Could you check a few things on this model? Use its own coordinates, in mm. A direction names the side the tool comes from. Coordinates: 2 decimals unless noted, no trailing zeros. Loops run counter-clockwise (first coordinate to the right, second up) from the corner with the lowest first, then second, coordinate; pieces in that order, holes last. Notation, with made-up numbers: (-6, 84.25) - (39, 84.25) arc R20 ccw to (39, 93.25) - close; hole circle Ø5 at (32, -15.75). An arc over 180 degrees is marked (long way). One line per question, with ' | ' between items. Start each with the question number.
1. Please list where these lines run through material, in increasing order: L1, parallel to Z at x = 0, y = 7.25; L2, parallel to Y at x = 0, z = 10.5; L3, parallel to Z at x = -1, y = 6. Write a range as [from, to].
2. Which directions (+Z, -Z, +X, -X, +Y, -Y) give clear straight access to the entire face, cutting with the end or side of a thin tool? Please do faces 1 (the cylindrical face through (1.43, -6.15, 19.45)), 2 (the cylindrical face through (3.958, 1.247, 19.591)).
3. I want a section at A-A, the plane y = 0. Write out the boundary of the cut face in (x, z), then the cut area to 3 significant figures.
4. I want a section at C-C, the plane z = 7. Write out the boundary of the cut face in (x, y), then the cut area to 3 significant figures.
5. I want a section at D-D, the plane y = 3. Write out the boundary of the cut face in (x, z), then the cut area to 3 significant figures.
6. I want a section at B-B, the plane x = 0. Write out the boundary of the cut face in (y, z).
7. We'd pull the mould along Z, two halves only. Please class faces 3 (the flat face through (2, -2, 13)), 4 (the cylindrical face through (-1.5, 5.17, 7.07)), 5 (the flat face through (2, -2, 0)): pulls with the +Z half, pulls with the -Z half, needs draft (parallel to the pull), parting line crosses it, or undercut.
8. I'm going to push flat-ended pins straight in: P1, Ø10, axis at x = 6.5, z = 14, coming from the -Y side; P2, Ø1, axis at x = -1, z = 22.5, coming from the +Y side; P3, Ø4, axis at y = 2.5, z = 13.5, coming from the +X side. Where does each tip first touch, or does it pass through?
from build123d import *

# Parameters (mm, degrees)
F0_R          = 8.5
F0_R_2        = 2.45
F1_DEPTH      = 26
F2_R          = 4.15
F2_R_2        = 2.45
F3_DEPTH      = 13
F4_R          = 1.5
F5_DEPTH      = 25
F5_DEPTH_BACK = 25


with BuildPart() as f1:
    # F0 (on Top) → F1 (new body)
    with BuildSketch(Plane.XY):
        Circle(F0_R)
        Circle(F0_R_2, mode=Mode.SUBTRACT)
    extrude(amount=F1_DEPTH)

    # F2 (on face) → F3 (cut)
    with BuildSketch(Plane.XY.offset(26)):
        Circle(F2_R)
        Circle(F2_R_2, mode=Mode.SUBTRACT)
    extrude(amount=-F3_DEPTH, mode=Mode.SUBTRACT)

    # F4 (on Front) → F5 (cut, two sides)
    with BuildSketch(Plane.XZ) as f5_sk:
        with Locations((0, 19)):
            Circle(F4_R)
        with Locations((0, 7)):
            Circle(F4_R)
    extrude(amount=-F5_DEPTH, mode=Mode.SUBTRACT)
    extrude(f5_sk.sketch, amount=F5_DEPTH_BACK, mode=Mode.SUBTRACT)


solid = f1.part
Results are:
1) L1: z = [0, 5.5], [8.5, 17.5], [20.5, 26] | L2: y = [-8.5, -2.45], [2.45, 8.5] | L3: z = [0, 5.88], [8.12, 17.88], [20.12, 26]
2) face 1: +Y, -Y | face 2: +Z
3) outline: (-8.5, 0) - (-2.45, 0) - (-2.45, 13) - (-4.15, 13) - (-4.15, 26) - (-8.5, 26) - close; (2.45, 0) - (8.5, 0) - (8.5, 26) - (4.15, 26) - (4.15, 13) - (2.45, 13) - close | area: 270 mm2
4) outline: (-1.5, -8.37) - (-1.5, -1.94) arc R2.45 cw to (-1.5, 1.94) - (-1.5, 8.37) arc R8.5 ccw to start; (1.5, -8.37) arc R8.5 ccw to (1.5, 8.37) - (1.5, 1.94) arc R2.45 cw to (1.5, -1.94) - close | area: 171 mm2
5) outline: (-7.95, 0) - (7.95, 0) - (7.95, 26) - (2.87, 26) - (2.87, 13) - (-2.87, 13) - (-2.87, 26) - (-7.95, 26) - close; hole circle Ø3 at (0, 7) | area: 332 mm2
6) outline: (-8.5, 0) - (-2.45, 0) - (-2.45, 5.5) - (-8.5, 5.5) - close; (-8.5, 8.5) - (-2.45, 8.5) - (-2.45, 13) - (-4.15, 13) - (-4.15, 17.5) - (-8.5, 17.5) - close; (-8.5, 20.5) - (-4.15, 20.5) - (-4.15, 26) - (-8.5, 26) - close; (2.45, 0) - (8.5, 0) - (8.5, 5.5) - (2.45, 5.5) - close; (2.45, 8.5) - (8.5, 8.5) - (8.5, 17.5) - (4.15, 17.5) - (4.15, 13) - (2.45, 13) - close; (4.15, 20.5) - (8.5, 20.5) - (8.5, 26) - (4.15, 26) - close
7) face 3: pulls with the +Z half | face 4: undercut | face 5: pulls with the -Z half
8) P1: stops at y = -8.37 | P2: stops at y = 8.49 | P3: stops at x = 8.49
